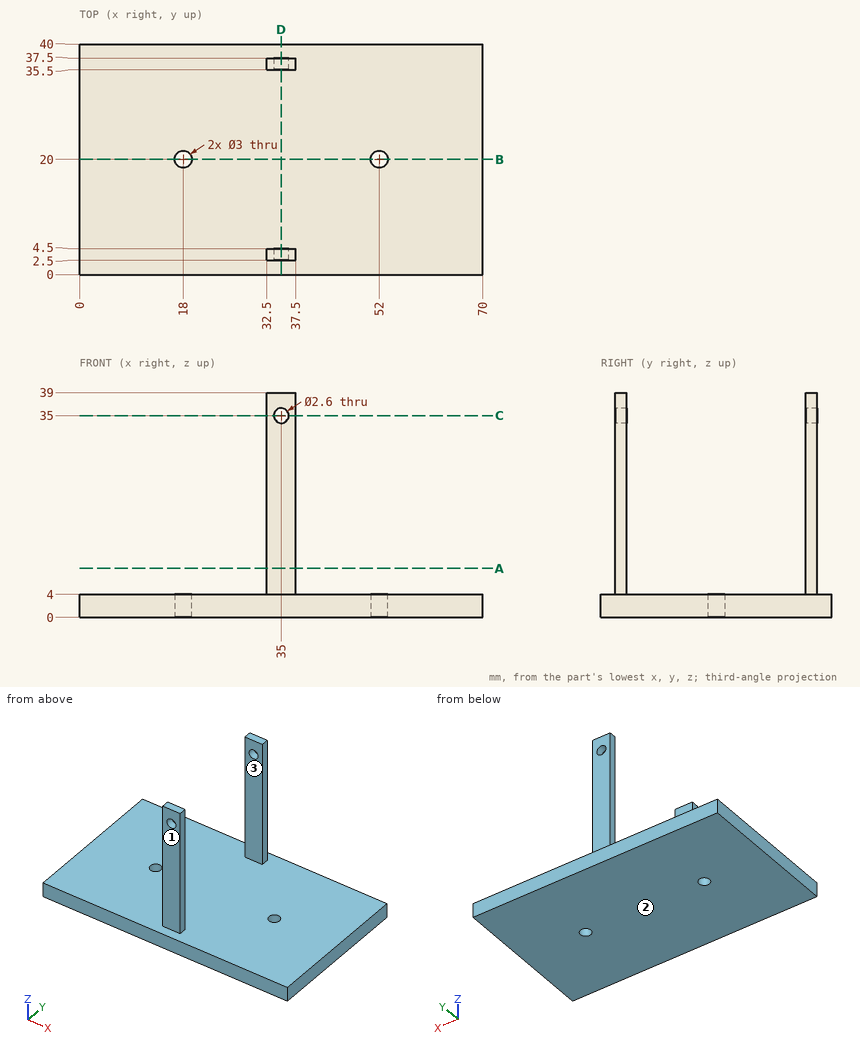
Can you work these out from the drawing? Everything is in mm from the part's minimum corner. Coordinates: 2 decimals unless noted, no trailing zeros. Loops run counter-clockwise (first coordinate to the right, second up) from the corner with the lowest first, then second, coordinate; pieces in that order, holes last. Notation, with made-up numbers: (-34.5, -15) - (13.5, -15) arc R22 ccw to (13.5, 23) - close; hole circle Ø5 at (-31.75, 14). An arc over 180 degrees is marked (long way). Use a Markdown table: item, result.
Item 1: I want a section at B-B on y = 20. Please give me the cut outline in (x, z).
Numbers:
| item | result |
|---|---|
| outline | (0, 0) - (16.5, 0) - (16.5, 4) - (0, 4) - close; (19.5, 0) - (50.5, 0) - (50.5, 4) - (19.5, 4) - close; (53.5, 0) - (70, 0) - (70, 4) - (53.5, 4) - close |
Item 2: Will these pins go through, and if not, where does the flat tip stop? pin 1 (1.6 mm diameter, centred on y = 3, z = 13.5, fed in from -X); pin 2 (20 mm diameter, centred on x = 38.5, y = 20, fed in from +Z); pin 3 (6 mm diameter, centred on x = 58.5, y = 26, fed in from -Z); pin 4 (0.6 mm diameter, centred on y = 36, z = 17.5, fed in from +X).
Numbers:
| item | result |
|---|---|
| pin 1 | stops at x = 32.5 |
| pin 2 | stops at z = 4 |
| pin 3 | stops at z = 0 |
| pin 4 | stops at x = 37.5 |
Item 3: I want a section at C-C on z = 35. Please give me the cut outline in (x, y).
Numbers:
| item | result |
|---|---|
| outline | (32.5, 2.5) - (33.7, 2.5) - (33.7, 4.5) - (32.5, 4.5) - close; (32.5, 35.5) - (33.7, 35.5) - (33.7, 37.5) - (32.5, 37.5) - close; (36.3, 2.5) - (37.5, 2.5) - (37.5, 4.5) - (36.3, 4.5) - close; (36.3, 35.5) - (37.5, 35.5) - (37.5, 37.5) - (36.3, 37.5) - close |
Item 4: We'd pull the mould along Y, two halves only. Please class the marked faces 1, 2 and 3: released by +Y, released by -Y, zero draft, split by the parting line, or undercut.
Numbers:
| item | result |
|---|---|
| face 1 | released by -Y |
| face 2 | zero draft |
| face 3 | undercut |
Item 5: I want a section at A-A on z = 8.5. Please give me the cut outline in (x, y), and give its area (3 significant figures).
Numbers:
| item | result |
|---|---|
| outline | (32.5, 2.5) - (37.5, 2.5) - (37.5, 4.5) - (32.5, 4.5) - close; (32.5, 35.5) - (37.5, 35.5) - (37.5, 37.5) - (32.5, 37.5) - close |
| area | 20.0 mm2 |
Item 6: If I drill on probe 1 along X at (y, z) = (20, 2); probe 2 along Z at (x, y) = (35, 35.9); probe 3 along Y at (x, z) = (52, 1.8), over which ranges is the centre line in solid material (lowest first)? Write a range as from..to.
Numbers:
| item | result |
|---|---|
| probe 1 | x = 0..16.5, 19.5..50.5, 53.5..70 |
| probe 2 | z = 0..33.7, 36.3..39 |
| probe 3 | y = 0..18.5, 21.5..40 |
Item 7: I want a section at D-D on x = 35. Please give me the cut outline in (y, z).
Numbers:
| item | result |
|---|---|
| outline | (0, 0) - (40, 0) - (40, 4) - (37.5, 4) - (37.5, 33.7) - (35.5, 33.7) - (35.5, 4) - (4.5, 4) - (4.5, 33.7) - (2.5, 33.7) - (2.5, 4) - (0, 4) - close; (2.5, 36.3) - (4.5, 36.3) - (4.5, 39) - (2.5, 39) - close; (35.5, 36.3) - (37.5, 36.3) - (37.5, 39) - (35.5, 39) - close |
